Read the model definition and answer for the solid it produces. Units are mm, in the model's axes. A direction names the side the tool comes from. Give positions to 0.01 mm unless a question says otherwise; leave off trailing zeros. Write each loop counter-clockwise with the first axis right and the second up, starting at its lowest first coordinate (ties: lowest second). Pieces come first, ordered by that corner, then holes. Notation, with made-up numbers: (17.25, -34.5) -> (24.25, -34.5) arc R11 cw to (24.25, -16.5) -> close; hole circle Ø5 at (36, -21). An arc over 180 degrees is marked (long way). Answer as CSV lines item,"result". Start each with the question number.
1. The part is cut by section A-A, the plane z = 11. Determine the outline of the cut face in (x, y).
2. The part is cut by section D-D, the plane z = -11. Determine the outline of the cut face in (x, y).
3. Find the intervals of material crossed by line 1 (X direction, y = -4.5, z = -5.75); line 2 (X direction, y = 3, z = 11.5); line 3 (Y direction, x = -54.35, z = 11), in increasing order.
4. The part is cut by section C-C, the plane y = -5.2. Determine the outline of the cut face in (x, z).
5. A tool of negligible diameter and unlimited length cuts with its end or side. For faces 1 (the cylindrical face through (44.714, 2.958, 11.325)), 2 (the flat face through (-1, 0, 0)), 3 (the cylindrical face through (54.28, -4.19, -6.39)), from which of +Z, -Z, +X, -X, +Y, -Y can it reach the whole face along a straight path? Write none if from no direction.
6. The part is cut by section B-B, the plane x = 43.25. Determine the outline of the cut face in (y, z), and give its area (3 significant figures).
7. For a pull along Y with two mould halves and no side action, classify faces 4 (the cylindrical face through (-54.2, -4.3, -9.8)), 5 (the flat face through (52.25, -5, 0)), 6 (the flat face through (54, -11, 0)), 7 (the flat face through (1, 6, 0)) as pulls with the +Y half, pulls with the -Y half, needs draft (parallel to the pull), parting line crosses it, or undercut.
from build123d import *

# Parameters (mm, degrees)
SKETCH_1_W      = 104.5
SKETCH_1_H      = 30
SKETCH_1_R      = 1.5
EXTRUDE_1_DEPTH = 6
SKETCH_2_W      = 30
SKETCH_2_H      = 17
SKETCH_2_R      = 1.5
EXTRUDE_2_DEPTH = 4
EXTRUDE_START   = 4
SKETCH_3_W      = 30
SKETCH_3_H      = 17
SKETCH_3_R      = 1.5
EXTRUDE_3_DEPTH = 4


with BuildPart() as part:
    # 草图1 → 凸台-拉伸1 (new body)
    with BuildSketch(Plane(origin=(0, 0, 0), x_dir=(1, 0, 0), z_dir=(0, 1, 0))):
        Rectangle(SKETCH_1_W, SKETCH_1_H)
        with Locations(Location((-31.75, 11, 0), (0, 0, 270))):
            Circle(SKETCH_1_R, mode=Mode.SUBTRACT)
        with Locations(Location((43.25, 11, 0), (0, 0, 270))):
            Circle(SKETCH_1_R, mode=Mode.SUBTRACT)
        with Locations(Location((43.25, -11, 0), (0, 0, 90))):
            Circle(SKETCH_1_R, mode=Mode.SUBTRACT)
        with Locations(Location((-31.75, -11, 0), (0, 0, 90))):
            Circle(SKETCH_1_R, mode=Mode.SUBTRACT)
    extrude(amount=EXTRUDE_1_DEPTH)

    # 草图2 → 凸台-拉伸2 (add)
    with BuildSketch(Plane.ZY.offset(52.25)):
        with Locations((0, -2.5)):
            Rectangle(SKETCH_2_W, SKETCH_2_H)
        with Locations((11, -5.2)):
            Circle(SKETCH_2_R, mode=Mode.SUBTRACT)
        with Locations(Location((-11, -5.2, 0), (0, 0, 180))):
            Circle(SKETCH_2_R, mode=Mode.SUBTRACT)
    extrude(amount=EXTRUDE_2_DEPTH)

    # 草图3 → 凸台-拉伸3 (add)
    with BuildSketch(Plane(origin=(52.25, 0, 0), x_dir=(0, 0, -1), z_dir=(1, 0, 0)).offset(EXTRUDE_START)):
        with Locations((0, -2.5)):
            Rectangle(SKETCH_3_W, SKETCH_3_H)
        with Locations(Location((-11, -5.2, 0), (0, 0, 180))):
            Circle(SKETCH_3_R, mode=Mode.SUBTRACT)
        with Locations((7.5, -5.2)):
            Circle(SKETCH_3_R, mode=Mode.SUBTRACT)
    extrude(amount=-EXTRUDE_3_DEPTH)


solid = part.part
Results found:
1,outline,"(-56.25, -11) -> (-52.25, -11) -> (-52.25, -6.7) -> (-56.25, -6.7) -> close; (-56.25, -3.7) -> (-52.25, -3.7) -> (-52.25, 0) -> (-33.25, 0) -> (-33.25, 6) -> (-56.25, 6) -> close; (-30.25, 0) -> (41.75, 0) -> (41.75, 6) -> (-30.25, 6) -> close; (44.75, 0) -> (52.25, 0) -> (52.25, -3.7) -> (56.25, -3.7) -> (56.25, 6) -> (44.75, 6) -> close; (52.25, -11) -> (56.25, -11) -> (56.25, -6.7) -> (52.25, -6.7) -> close"
2,outline,"(-56.25, -11) -> (-52.25, -11) -> (-52.25, -6.7) -> (-56.25, -6.7) -> close; (-56.25, -3.7) -> (-52.25, -3.7) -> (-52.25, 0) -> (-33.25, 0) -> (-33.25, 6) -> (-56.25, 6) -> close; (-30.25, 0) -> (41.75, 0) -> (41.75, 6) -> (-30.25, 6) -> close; (44.75, 0) -> (52.25, 0) -> (52.25, -11) -> (56.25, -11) -> (56.25, 6) -> (44.75, 6) -> close"
3,line 1,"x = -56.25 to -52.25, 52.25 to 56.25"
3,line 2,"x = -56.25 to -33.16, -30.34 to 41.84, 44.66 to 56.25"
3,line 3,"y = -11 to -6.7, -3.7 to 6"
4,outline,"(-56.25, -15) -> (-52.25, -15) -> (-52.25, -12.5) -> (-56.25, -12.5) -> close; (-56.25, -9.5) -> (-52.25, -9.5) -> (-52.25, 9.5) -> (-56.25, 9.5) -> close; (-56.25, 12.5) -> (-52.25, 12.5) -> (-52.25, 15) -> (-56.25, 15) -> close; (52.25, -15) -> (56.25, -15) -> (56.25, -9) -> (52.25, -9) -> close; (52.25, -6) -> (56.25, -6) -> (56.25, 9.5) -> (52.25, 9.5) -> close; (52.25, 12.5) -> (56.25, 12.5) -> (56.25, 15) -> (52.25, 15) -> close"
5,face 1,"+Y, -Y"
5,face 2,"+Z, -Z, -Y"
5,face 3,"+X"
6,outline,"(0, -15) -> (6, -15) -> (6, -12.5) -> (0, -12.5) -> close; (0, -9.5) -> (6, -9.5) -> (6, 9.5) -> (0, 9.5) -> close; (0, 12.5) -> (6, 12.5) -> (6, 15) -> (0, 15) -> close"
6,area,"144 mm²"
7,face 4,"undercut"
7,face 5,"needs draft"
7,face 6,"pulls with the -Y half"
7,face 7,"pulls with the +Y half"
